from build123d import *

# Parameters (mm, degrees)
F2_SIZE = 2


with BuildPart() as f1:
    # F0 (on Front) → F1 (revolve)
    with BuildSketch(Plane.XZ):
        with BuildLine():
            Line((0, 32.5), (0, 27.5))
            Line((0, 27.5), (13, 27.5))
            Line((13, 27.5), (13, 22.205228))
            Line((13, 22.205228), (41, 25))
            Line((41, 25), (41, 32.5))
            Line((41, 32.5), (34, 32.5))
            ThreePointArc((34, 32.5), (31.87868, 33.37868), (31, 35.5))
            Line((31, 35.5), (31, 62))
            ThreePointArc((31, 62), (31.87868, 64.12132), (34, 65))
            Line((34, 65), (41, 65))
            Line((41, 65), (41, 75))
            Line((41, 75), (36, 75))
            Line((36, 75), (36, 70))
            Line((36, 70), (31, 70))
            Line((31, 70), (31, 75))
            Line((31, 75), (23, 75))
            Line((23, 75), (23, 70))
            Line((23, 70), (18, 70))
            Line((18, 70), (18, 75))
            Line((18, 75), (8, 75))
            Line((8, 75), (8, 70))
            Line((8, 70), (5, 70))
            Line((5, 70), (5, 75))
            Line((5, 75), (0, 75))
            Line((0, 75), (0, 65))
            Line((0, 65), (7, 65))
            ThreePointArc((7, 65), (9.12132, 64.12132), (10, 62))
            Line((10, 62), (10, 35.5))
            ThreePointArc((10, 35.5), (9.12132, 33.37868), (7, 32.5))
            Line((7, 32.5), (0, 32.5))
        make_face()
    revolve(axis=Axis((20.5, 0, 0), (1, 0, 0)))

    # F2
    f2_edges = [f1.edges().sort_by_distance(p)[0] for p in [
        (41, 0, -75),
        (0, 0, -75),
    ]]
    chamfer(f2_edges, length=F2_SIZE)


solid = f1.part
Check sheet for the modelled part. Datum: model origin and axes. Units: mm. A direction names the side the tool comes from. Give positions to 0.01 mm unless a question says otherwise; leave off trailing zeros. Loops run counter-clockwise (first coordinate to the right, second up) from the corner with the lowest first, then second, coordinate; pieces in that order, holes last. Notation, with made-up numbers: M -32,76.25 L 1,76.25 A23 ccw 1,111.25 Z; hole C 41.25,66 d6. An arc over 180 degrees is marked long. Answer as a JSON object with one key per item and string values. Group by question number.
Q1. Release check for a two-part mould opening along X. For faces 6 (the flat face through (8, 50, 50)), 7 (the conical face through (40.875, -72.503, -9.519)), 8 (the flat face through (5, 50, -50)), 9 (the cylindrical face through (37.55, -19.52, 62)) record: released by +X, released by -X, zero draft, split by the parting line, or undercut.
Q2. Material ranges on line 1 along Z through (x, y) = (4.25, 0); line 2 along Y through (x, z) = (7, 0), recorded low to high. Write a range as [from, to].
Q3. Go/stop test with flat-tipped pins: P1, Ø1, axis at x = 25, z = -22.5, coming from the +Y side; P2, Ø12, axis at x = 11, y = -43, coming from the -Z side; P3, Ø6, axis at y = -14, z = 34, coming from the +X side; P4, Ø10, axis at y = -22, z = -24, coming from the -X side. Record where each tip stops, or that it passes through.
Q4. Cross-section at A-A on x = 27.5. Record the cut outline in (y, z), then the cut area to 3 significant figures.
Q5. Access from +Z, -Z, +X, -X, +Y, -Y to the whole of each face (thin tool, end or side, straight path). Record for faces 1 (the flat face through (31, 27, -27)), 2 (the flat face through (0, -7, -27)), 3 (the flat face through (36, 50, 50)), 4 (the cylindrical face through (12.93, -74.362, -9.764)), 5 (the cylindrical face through (6.591, 26.846, -5.961)).
Evaluation:
{
 "1": {"face 6": "undercut", "face 7": "released by +X", "face 8": "undercut", "face 9": "zero draft"},
 "2": {"line 1": "z = [-75, -65], [-32.5, -27.5], [27.5, 32.5], [65, 75]", "line 2": "y = [-70, -65], [-32.5, -27.5], [27.5, 32.5], [65, 70]"},
 "3": {"P1": "stops at y = 71.7", "P2": "stops at z = -65.24", "P3": "stops at x = 31.55", "P4": "stops at x = 0"},
 "4": {"outline": "C 0,0 d150; hole C 0,0 d47.31", "area": "15,900 mm2"},
 "5": {"face 1": "+X", "face 2": "+Z, -Z, -X, +Y, -Y", "face 3": "none", "face 4": "+X, -X", "face 5": "-X"}
}
